The figure shows three views and two pictorial views of one solid part (mm, origin at its lowest corner). Answer the questions. Give positions to 0.01 mm unless a question says otherwise; leave off trailing zeros. Loops run counter-clockwise (first coordinate to the right, second up) from the corner with the lowest first, then second, coordinate; pieces in that order, holes last. Notation, with made-up numbers: (77.25, 45) - (121.25, 45) arc R16 cw to (121.25, 72) - close; hole circle Ø10 at (63, 46.25). An arc over 180 degrees is marked (long way). Write item = value, one per line.
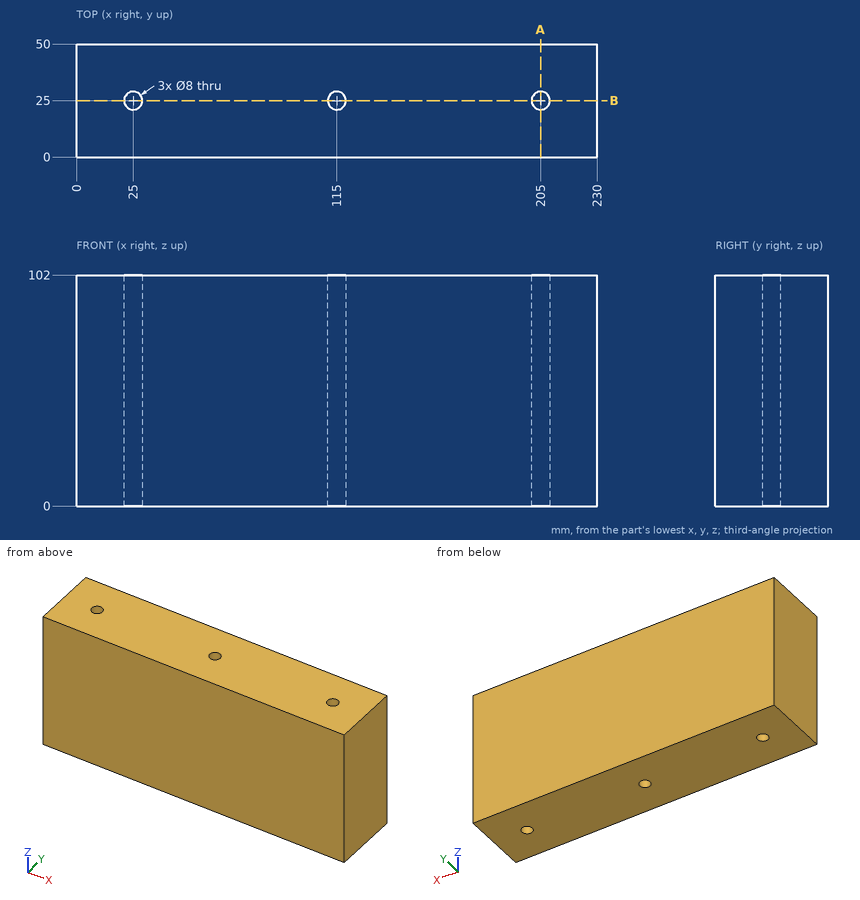
1) Find the intervals of material crossed by probe 1 along Y at (x, z) = (25, 28); probe 2 along X at (y, z) = (26.5, 14); probe 3 along X at (y, z) = (22.5, 44), in increasing order.
Output:
probe_1 = 0 to 21, 29 to 50
probe_2 = 0 to 21.29, 28.71 to 111.29, 118.71 to 201.29, 208.71 to 230
probe_3 = 0 to 21.88, 28.12 to 111.88, 118.12 to 201.88, 208.12 to 230
2) A cutting plane is placed at A-A on x = 205. Determine the outline of the cut face in (y, z), then the cut area to 3 significant figures.
Output:
outline = (0, 0) - (21, 0) - (21, 102) - (0, 102) - close; (29, 0) - (50, 0) - (50, 102) - (29, 102) - close
area = 4,280 mm²
3) This flat-tipped pin is pushed along its axis until it touches: P1, Ø6.5, axis at x = 115, y = 25, coming from the -Z side. Where does it stop, or does it pass through?
Output:
P1 = through
4) A cutting plane is placed at B-B on y = 25. Determine the outline of the cut face in (x, z), then the cut area to 3 significant figures.
Output:
outline = (0, 0) - (21, 0) - (21, 102) - (0, 102) - close; (29, 0) - (111, 0) - (111, 102) - (29, 102) - close; (119, 0) - (201, 0) - (201, 102) - (119, 102) - close; (209, 0) - (230, 0) - (230, 102) - (209, 102) - close
area = 21,000 mm²
